Can you work these out from the model? Positions are in its coordinate system, mm. Face numbers are marked on the shaded views. A direction names the side the tool comes from. Coordinates: 2 decimals unless noted, no trailing zeros. Loops run counter-clockwise (first coordinate to the right, second up) from the corner with the lowest first, then second, coordinate; pieces in that order, holes last. Notation, with made-up numbers: M -32,80.5 L 3,80.5 A18 cw 3,100.5 Z; hole C -15,65 d11. An arc over 180 degrees is marked long. Return JSON: item names as keys, results as strings. Group by question number.
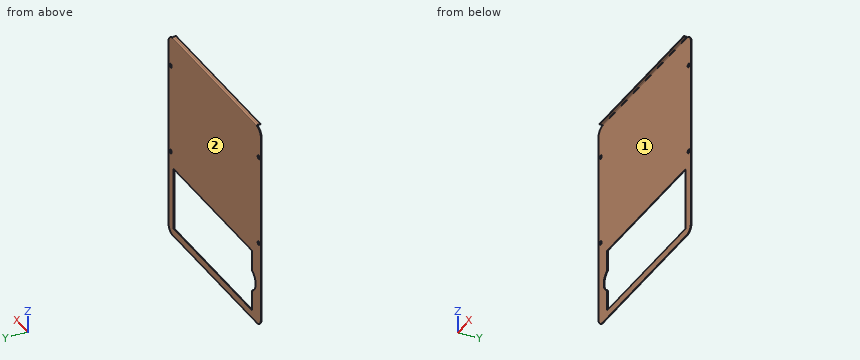
```python
from build123d import *

# Parameters (mm, degrees)
BASE_FLANGE1_DEPTH      = 114.5
BASE_FLANGE1_DEPTH_BACK = 114.5
SKETCH1_W               = 264
SKETCH1_H               = 0.8
FILLET1_R               = 10
EDGE_FLANGE2_DEPTH      = 209
SKETCH14_R              = 2.45
CUT_EXTRUDE1_DEPTH      = 176.961710436
CUT_EXTRUDE2_DEPTH      = 176.961710436


# Sheet-metal steps are written as plain solids
with BuildPart() as part:
    # Sketch1 → Base-Flange1 (new, two sides: drawn at the far end of the back side and taken through both)
    with BuildSketch(Plane(origin=(0, 0, 0), x_dir=(0, 0, -1), z_dir=(1, 0, 0)).offset(-BASE_FLANGE1_DEPTH_BACK)):
        with Locations((0, -0.4)):
            Rectangle(SKETCH1_W, SKETCH1_H)
    extrude(amount=BASE_FLANGE1_DEPTH + BASE_FLANGE1_DEPTH_BACK)

    # Fillet1
    fillet1_edges = [part.edges().sort_by_distance(p)[0] for p in [
        (-114.5, -0.4, 132),
        (-114.5, -0.4, -132),
        (114.5, -0.4, 132),
        (114.5, -0.4, -132),
    ]]
    fillet(fillet1_edges, radius=FILLET1_R)

    # Edge-Flange2 section (across the edge) → Edge-Flange2 (add)
    with BuildSketch(Plane(origin=(104.5, -0.8, 132.7366), x_dir=(0, 0, -1), z_dir=(-1, 0, 0))):
        with BuildLine():
            Line((-0.8, 0.7366), (-0.8, 3.7))
            Line((-0.8, 3.7), (0, 3.7))
            Line((0, 3.7), (0, 0.7366))
            ThreePointArc((0, 0.7366), (0.215745145, 0.215745145), (0.7366, 0))
            Line((0.7366, 0), (0.7366, -0.8))
            ThreePointArc((0.7366, -0.8), (-0.34994028, -0.34994028), (-0.8, 0.7366))
        make_face()
    extrude(amount=EDGE_FLANGE2_DEPTH)

    # Sketch14 → Cut-Extrude1 (cut, through all)
    with BuildSketch(Plane(origin=(0, 0, 0), x_dir=(1, 0, 0), z_dir=(0, 1, 0))):
        with Locations(Location((-109, -92.5, 0), (0, 0, 270))):
            Circle(SKETCH14_R)
        with Locations(Location((-109, 22.5, 0), (0, 0, 270))):
            Circle(SKETCH14_R)
    cut_extrude1 = extrude(amount=-CUT_EXTRUDE1_DEPTH, mode=Mode.SUBTRACT)

    # Mirror1: Cut-Extrude1 across plane
    add(cut_extrude1.mirror(Plane(origin=(0, 0, 0), x_dir=(0, 0, 1), z_dir=(1, 0, 0))), mode=Mode.SUBTRACT)

    # Sketch15 → Cut-Extrude2 (cut, through all)
    with BuildSketch(Plane(origin=(0, 0, 0), x_dir=(1, 0, 0), z_dir=(0, 1, 0))):
        with BuildLine():
            Line((-93, 121.85), (101.5, 121.85))
            Line((101.5, 121.85), (101.5, 41.85))
            Line((101.5, 41.85), (-93, 41.85))
            Line((-93, 41.85), (-93, 68.9))
            ThreePointArc((-93, 68.9), (-101.5, 81.85), (-93, 94.8))
            Line((-93, 94.8), (-93, 121.85))
        make_face()
    extrude(amount=-CUT_EXTRUDE2_DEPTH, mode=Mode.SUBTRACT)


solid = part.part
```
1) For pin 1 (1.7 mm diameter, centred on y = -2.5, z = 133, fed in from -X); pin 2 (3 mm diameter, centred on x = 38.5, z = 29.5, fed in from -Y); pin 3 (1.7 mm diameter, centred on y = -2, z = 133, fed in from +X), each with a flat end and sliding along its axis, tell me the tip position at first contact or that it passes through.
2) For the marked faces 1 and 2, which set-ups out of +Z, -Z, +X, -X, +Y, -Y let a thin tool reach every point of the face, with its end or its side?
3) If I drill on line 1 (X direction, y = -0.25, z = 92.5); line 2 (Z direction, x = 109, y = -0.35); line 3 (Y direction, x = 23, z = 109), over which ranges is the centre line in solid material (lowest first)? Write a range as from..to.
4) Suppose I cut it at A-A, the plane x = -40.5. List the corners of the cut face in (y, z) for me.
5) Suppose I cut it at B-B, the plane z = 105.5. List the corners of the cut face in (x, y) for me, then the cut area to 3 significant figures.
Returned:
{
 "1": {"pin 1": "stops at x = -104.5", "pin 2": "stops at y = -0.8", "pin 3": "stops at x = 104.5"},
 "2": {"face 1": "-Z, +X, -X, -Y", "face 2": "+Z, -Z, +X, -X, +Y"},
 "3": {"line 1": "x = -114.5..-111.45, -106.55..106.55, 111.45..114.5", "line 2": "z = -130.93..-24.95, -20.05..90.05, 94.95..130.93", "line 3": "y = -0.8..0"},
 "4": {"outline": "M -4.5,132.74 L -1.54,132.74 A0.74 cw -0.8,132 L -0.8,-41.85 L 0,-41.85 L 0,132 A1.54 ccw -1.54,133.54 L -4.5,133.54 Z; M -0.8,-132 L 0,-132 L 0,-121.85 L -0.8,-121.85 Z"},
 "5": {"outline": "M -114.5,-0.8 L 114.5,-0.8 L 114.5,0 L -114.5,0 Z", "area": "183 mm²"}
}
